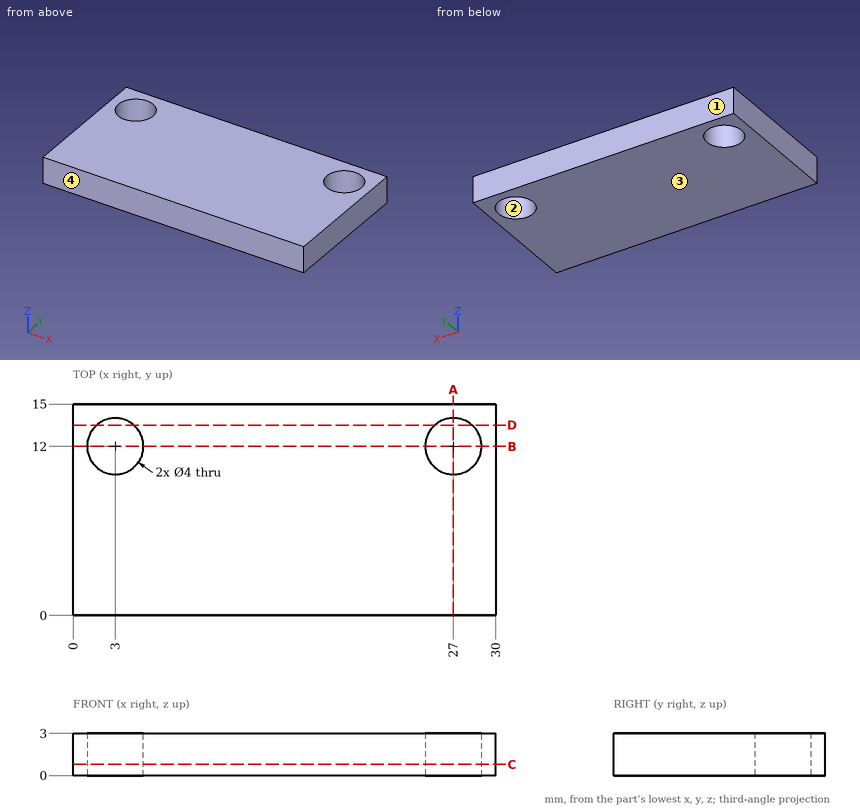
Verification items for this drawing (mm, ordinates from the low corner). Give positions to 0.01 mm unless a question says otherwise; leave off trailing zeros. Loops run counter-clockwise (first coordinate to the right, second up) from the corner with the lowest first, then second, coordinate; pieces in that order, holes last. Notation, with made-up numbers: M 61.5,24 L 90.5,24 A17 ccw 90.5,51 Z; hole C -2,-31.75 d2. An arc over 180 degrees is marked long. Return JSON: item names as keys, results as strings. Group by question number.
1. Thickness scan on L1, parallel to Y at x = 27, z = 0.9; L2, parallel to X at y = 10.5, z = 1.5; L3, parallel to X at y = 13, z = 0.9. Record the ranges inside material, lowest first.
2. Cross-section at A-A on x = 27. Record the boundary of the cut face in (y, z).
3. Cross-section at B-B on y = 12. Record the boundary of the cut face in (x, z), plus the area to 3 significant figures.
4. Mould release check, pull along Y, two halves, no side actions. Record for the marked faces 1, 2, 3 and 4: released by +Y, released by -Y, zero draft, split by the parting line, or undercut.
5. Go/stop test with a flat-tipped pin: pin 1 (3 mm diameter, centred on x = 27, y = 12, fed in from +Z). Record where the tip stops, or that it passes through.
6. Cross-section at C-C on z = 0.8. Record the boundary of the cut face in (x, y).
7. Cross-section at D-D on y = 13.5. Record the boundary of the cut face in (x, z), plus the area to 3 significant figures.
Return value:
{
 "1": {"L1": "0 to 10, 14 to 15", "L2": "0 to 1.68, 4.32 to 25.68, 28.32 to 30", "L3": "0 to 1.27, 4.73 to 25.27, 28.73 to 30"},
 "2": {"outline": "M 0,0 L 10,0 L 10,3 L 0,3 Z; M 14,0 L 15,0 L 15,3 L 14,3 Z"},
 "3": {"outline": "M 0,0 L 1,0 L 1,3 L 0,3 Z; M 5,0 L 25,0 L 25,3 L 5,3 Z; M 29,0 L 30,0 L 30,3 L 29,3 Z", "area": "66.0 mm^2"},
 "4": {"face 1": "released by +Y", "face 2": "undercut", "face 3": "zero draft", "face 4": "released by -Y"},
 "5": {"pin 1": "through"},
 "6": {"outline": "M 0,0 L 30,0 L 30,15 L 0,15 Z; hole C 3,12 d4; hole C 27,12 d4"},
 "7": {"outline": "M 0,0 L 1.68,0 L 1.68,3 L 0,3 Z; M 4.32,0 L 25.68,0 L 25.68,3 L 4.32,3 Z; M 28.32,0 L 30,0 L 30,3 L 28.32,3 Z", "area": "74.1 mm^2"}
}
